```python
from build123d import *

# Parameters (mm, degrees)
SKETCH_1_R          = 14.925
EXTRUDE_1_DEPTH     = 2
EXTRUDE_START       = -28
SKETCH_2_R          = 16.925
SKETCH_2_R_2        = 14.925
EXTRUDE_2_DEPTH     = 28
SKETCH_3_W          = 0.05
SKETCH_3_H          = 26
CUT_EXTRUDE_1_DEPTH = 27


with BuildPart() as part:
    # Эскиз1 → Бобышка-Вытянуть1 (new body)
    with BuildSketch(Plane.XY):
        Circle(SKETCH_1_R)
    extrude(amount=EXTRUDE_1_DEPTH)

    # Эскиз2 → Бобышка-Вытянуть2 (add)
    with BuildSketch(Plane.XY.offset(2).offset(EXTRUDE_START)):
        Circle(SKETCH_2_R)
        Circle(SKETCH_2_R_2, mode=Mode.SUBTRACT)
    extrude(amount=EXTRUDE_2_DEPTH)

    # Эскиз3 → Вырез-Вытянуть1 (cut)
    with BuildSketch(Plane(origin=(-4.399906999, 4.240400233, -22), x_dir=(1, 0, 0), z_dir=(0, 1, 0))):
        with Locations((4.39587448, -9.32957199)):
            Rectangle(SKETCH_3_W, SKETCH_3_H)
    extrude(amount=CUT_EXTRUDE_1_DEPTH, mode=Mode.SUBTRACT)


solid = part.part
```
For this review, take the finished solid that the model builds, in its own axes (mm). A direction names the side the tool comes from. Give positions to 0.01 mm unless a question says otherwise; leave off trailing zeros. Write each loop counter-clockwise with the first axis right and the second up, starting at its lowest first coordinate (ties: lowest second). Pieces come first, ordered by that corner, then holes.
Item 1: Insertion check: P1, Ø14, axis at y = 8.5, z = -8, coming from the +X side; P2, Ø3, axis at y = -7.5, z = -5.5, coming from the +X side; P3, Ø9, axis at x = -5.5, y = -3, coming from the -Z side. Each pin has a flat end and moves straight along its axis. Give the tip position at first contact, or say it passes through.
Item 2: Take a section at D-D (y = 12.5). Give the boundary of the cut face in (x, z), and give its area (3 significant figures).
Item 3: Wall thickness on probe 1 along Y at (x, z) = (0.5, -21.5); probe 2 along Z at (x, y) = (-10, 10); probe 3 along Y at (x, z) = (11.5, -11.75): over which ranges is each line inside the solid? List them lowest first.
Item 4: Take a section at C-C (z = -20.5). Give the boundary of the cut face in (x, y) (3 decimals), and give its area (3 significant figures).
Item 5: The part is to be moulded in two halves that separate along X. For faces 3 (the face through (13.787, -5.716, -13.182)), 4 (the face through (6, -14, -26)), 5 (the face through (16.143, 5.084, -12.196)), say which applies: +X half, -X half, draft (parallel to the pull), parting line (faces both ways), or undercut.
Item 6: Take a section at B-B (x = -10). Give the boundary of the cut face in (y, z), and give its area (3 significant figures).
Item 7: Machinability: for faces 1 (the face through (0, 0, 2)), 2 (the face through (0, 0, 0)), which of the approach directions +Z, -Z, +X, -X, +Y, -Y give a long, thin tool a straight path to every point of the face, cutting with its end or side? Answer none if there is none.
Item 8: Take a section at A-A (y = 0). Give the boundary of the cut face in (x, z) (3 decimals), and give its area (3 significant figures).
Established:
1. P1: stops at x = 16.86
1. P2: stops at x = 15.83
1. P3: stops at z = 0
2. outline: (-11.41, -26) - (-8.16, -26) - (-8.16, 0) - (-0.03, 0) - (-0.03, 0.33) - (0.02, 0.33) - (0.02, 0) - (8.16, 0) - (8.16, -26) - (11.41, -26) - (11.41, 2) - (-11.41, 2) - close
2. area: 215 mm2
3. probe 1: y = -16.92 to -14.92, 14.92 to 16.92
3. probe 2: z = 0 to 2
3. probe 3: y = -12.42 to -9.51, 9.51 to 12.42
4. outline: (-0.029, 14.925) - (-0.029, 16.925) arc R16.925 ccw (long way) to (0.021, 16.925) - (0.021, 14.925) arc R14.925 cw (long way) to start
4. area: 200 mm2
5. face 3: undercut
5. face 4: draft
5. face 5: parting line
6. outline: (-13.65, -26) - (-11.08, -26) - (-11.08, 0) - (11.08, 0) - (11.08, -26) - (13.65, -26) - (13.65, 2) - (-13.65, 2) - close
6. area: 189 mm2
7. face 1: +Z, +X, -X, +Y, -Y
7. face 2: -Z
8. outline: (-16.925, -26) - (-14.925, -26) - (-14.925, 0) - (14.925, 0) - (14.925, -26) - (16.925, -26) - (16.925, 2) - (-16.925, 2) - close
8. area: 172 mm2
